Design review of the part built by this model. Coordinates are the model's own, in mm. Coordinates: 2 decimals unless noted, no trailing zeros. Write each loop counter-clockwise with the first axis right and the second up, starting at its lowest first coordinate (ties: lowest second). Pieces come first, ordered by that corner, then holes. Notation, with made-up numbers: (-20.75, 58) - (-0.75, 58) arc R34 cw to (-0.75, 96) - close; hole circle Ø1 at (-4.5, -22.75). An arc over 180 degrees is marked (long way). Answer as a JSON object with one key per item and string values.
Autodesk Inventor part; units mm, degrees
ref_plane "YZ Plane" through (0, 0, 0) normal (1, 0, 0) x (0, 1, 0)
ref_plane "XZ Plane" through (0, 0, 0) normal (0, 1, 0) x (-1, 0, 0)
ref_plane "XY Plane" through (0, 0, 0) normal (0, 0, 1) x (1, 0, 0)
sketch "Sketch2" plane through (0, 0, 0) normal (1, 0, 0) x (0, 1, 0)
  line L0 (0, 0) -> (3.15, 0)
  line L1 (3.15, 0) -> (3.15, -4.9)
  line L2 (3.15, -4.9) -> (2.8, -4.9)
  line L3 (2.8, -4.9) -> (2.8, -20.5)
  line L4 (2.8, -20.5) -> (3.15, -20.5)
  line L5 (3.15, -20.5) -> (3.15, -25.4)
  line L6 (3.15, -25.4) -> (0, -25.4)
  line L7 (0, -25.4) -> (0, 0)
  dimension "d1" = 3.15
  dimension "d2" = 4.9
  dimension "d3" = 0.35
  dimension "d4" = 15.6
  dimension "d5" = 0.35
  dimension "d6" = 4.9
  dimension "d7" = 3.15
revolve "Revolution1" add sketch "Sketch2" angle 360 about axis through (0, 0, -25.4) along (0, 0, 1)
fillet "Fillet4" radius 0.4 2 edges at (0, -3.15, -25.4) (0, -3.15, 0)
fillet "Fillet5" radius 0.35 2 edges at (0, -3.15, -20.5) (0, -3.15, -4.9)
equation "\"d5\" = d3"
equation "\"d6\" = d2"
equation "\"d7\" = d1"
properties part number "Fusible de 13A"
(1) The part is to be moulded in two halves that separate along Z. For faces 1 (the face through (0.1, -2.8, -12.8)), 2 (the face through (-1.917, -2.5, -2.504)), 3 (the face through (0, 0, -25.4)), say which applies: pulls with the +Z half, pulls with the -Z half, needs draft (parallel to the pull), parting line crosses it, or undercut.
Solved:
{"face 1": "undercut", "face 2": "needs draft", "face 3": "pulls with the -Z half"}
(2) Take a section at C-C, the plane z = -12.25. Write out the cut boundary in (x, y).
Solved:
{"outline": "circle Ø5.6 at (0, 0)"}
(3) To check wall thickness, follow line 1 (Z direction, x = -1.75, y = 2.5); line 2 (Y direction, x = 0, z = -9); line 3 (Y direction, x = 2.5, z = -13.75). State the ranges of each line that lie inside material, in increasing order. Write a range as from..to.
Solved:
{"line 1": "z = -25.26..-20.61, -4.79..-0.14", "line 2": "y = -2.8..2.8", "line 3": "y = -1.26..1.26"}
